Can you work these out from the model? Positions are in its coordinate system, mm. Round coordinates to 2 decimals unless told otherwise and drop trailing zeros. Order: outer loops, then holes, each group sorted by start corner. A loop starts at its lowest first (then second) coordinate and runs counter-clockwise, first axis right, second up. Notation, with made-up numbers: M -10.75,14 L 22.25,14 A22 ccw 22.25,33 Z; hole C 65.5,63.25 d5. An arc over 180 degrees is marked long. Answer as a JSON object with one key per item and string values. Group by question number.
Autodesk Inventor part; units mm, degrees
ref_plane "Arbeitsebene4" through (0, 0, 3.25) normal (0, 0, 1) x (1, 0, 0)
ref_plane "YZ Plane" through (0, 0, 0) normal (1, 0, 0) x (0, 1, 0)
ref_plane "XZ Plane" through (0, 0, 0) normal (0, 1, 0) x (-1, 0, 0)
sketch "Skizze1" plane through (0, 0, 0) normal (0, 1, 0) x (-1, 0, 0)
  circle A0 centre (0, 0) radius 3.25
  dimension "d0" = 6.5
extrude "Extrusion1" add sketch "Skizze1" along normal blind 30
chamfer "Fasen1" distance 0.5 angle 45 2 edges at (3.25, 30, 0) (3.25, 0, 0)
ref_plane "Arbeitsebene4" through (0, 0, 3.25) normal (0, 0, 1) x (1, 0, 0)
sketch "Skizze4" plane through (0, 0, 3.25) normal (0, 0, 1) x (1, 0, 0)
  line L0 (-2.75, 30) -> (2.75, 30)
  point P0 (0, 0)
  point P1 (0, 4)
  point P2 (0, 26)
  dimension "d25" = 4
  dimension "d26" = 4
hole "Bohrung3" at (0, 4, 3.25) at (0, 26, 3.25) direction (0, 0, -1) diameter 2.5 end through all
properties part number "BMS_bolts_left" material "Edelstahl"
1) We'd pull the mould along X, two halves only. Please class faces 1 (the face through (0, 30, 0)), 2 (the face through (0.479, 24.845, -0.046)), 3 (the face through (0.705, 14.797, 3.173)): +X half, -X half, draft (parallel to the pull), parting line (faces both ways), or undercut.
2) If we section it at C-C on y = 15: Write out the boundary of the cut face in (x, z).
3) If we section it at D-D on x = -0.75: Count the separate pieces of the cut face and the enclosed holes in it, plus the area to 3 significant figures.
4) I need wall thicknesses on line 1 along Y through (x, z) = (0, 0); line 2 along Y through (x, z) = (-0.5, -1.5); line 3 along X through (y, z) = (26, -1.75). Which ranges of each line are inside material? Lowest first, please.
5) If we section it at A-A on z = 0: Write out the boundary of the cut face in (x, y), plus the area to 3 significant figures.
6) If we section it at B-B on y = 4: Write out the boundary of the cut face in (x, z), plus the area to 3 significant figures.
Findings:
{
 "1": {"face 1": "draft", "face 2": "undercut", "face 3": "parting line"},
 "2": {"outline": "C 0,0 d6.5"},
 "3": {"separate pieces": "3", "enclosed holes": "0", "area": "164 mm^2"},
 "4": {"line 1": "y = 0 to 2.75, 5.25 to 24.75, 27.25 to 30", "line 2": "y = 0 to 2.85, 5.15 to 24.85, 27.15 to 30", "line 3": "x = -2.74 to -1.25, 1.25 to 2.74"},
 "5": {"outline": "M -3.25,0.5 L -2.75,0 L 2.75,0 L 3.25,0.5 L 3.25,29.5 L 2.75,30 L -2.75,30 L -3.25,29.5 Z; hole C 0,4 d2.5; hole C 0,26 d2.5", "area": "185 mm^2"},
 "6": {"outline": "M -1.25,-3 L -1.25,3 A3.25 ccw Z; M 1.25,-3 A3.25 ccw 1.25,3 Z", "area": "17.3 mm^2"}
}
